Source: CAD feature listing. Evaluate the final solid. Frame: model axes, mm. A direction names the side the tool comes from. Give positions to 0.01 mm unless a question says otherwise; leave off trailing zeros. Order: outer loops, then holes, each group sorted by start corner. A loop starts at its lowest first (then second) coordinate and runs counter-clockwise, first axis right, second up.
from build123d import *

# Parameters (mm, degrees)
EXTRUDE_1_DEPTH        = 180
HOLE_WIZARD_M6_1_D     = 5
HOLE_WIZARD_M6_1_DEPTH = 28
HOLE_WIZARD_M6_1_TIP   = 1.502151548


with BuildPart() as part:
    # 草图1 → 凸台-拉伸1 (new body)
    with BuildSketch(Plane.XY):
        Polygon((12.5, 0), (0, 0), (-3.5, 3.5), (-3.5, 6.2), (2.25, 6.2), (2.25, 9.5), (10.25, 9.5), (10.25, 6.2), (16, 6.2), (16, 3.5), align=None)
    extrude(amount=EXTRUDE_1_DEPTH)

    # M6 螺纹孔1
    with Locations(Plane(origin=(6.25, 9.5, 158), x_dir=(0, 0, 1), z_dir=(0, 1, 0))):
        with Locations((0, 0), (-49, 0), (-136, 0), (-87, 0)):
            Hole(HOLE_WIZARD_M6_1_D / 2, depth=HOLE_WIZARD_M6_1_DEPTH)
            with Locations((0, 0, -(HOLE_WIZARD_M6_1_DEPTH + HOLE_WIZARD_M6_1_TIP / 2))):  # 118° drill point
                Cone(0, HOLE_WIZARD_M6_1_D / 2, HOLE_WIZARD_M6_1_TIP, mode=Mode.SUBTRACT)


solid = part.part
(1) Section A-A, the plane x = 6.25. Return loops of the section in (y, z).
(2) Section B-B, the plane z = 71. Return loops of the section in (x, y), plus the area to 4 significant figures.
(3) Access query for faces 1 (the flat face through (6, 9.5, 89)), 2 (the flat face through (-1, 6.2, 89)), 3 (the flat face through (10.25, 8, 89)). Directions: +Z, -Z, +X, -X, +Y, -Y. A direction counts if a zero-diameter tool reaches every point of the face in a straight line with its end or side. Return the directions, or none.
(4) Section D-D, the plane z = 154. Return loops of the section in (x, y).
(5) Line query: line 1 along Z through (x, y) = (6, 7.25); line 2 along X through (y, z) = (4.5, 158); line 3 along X through (y, z) = (7.75, 166). Output: solid intervals per line, ascending.
(6) Section C-C, the plane y = 1.5. Return loops of the section in (x, z), plus the area to 3 significant figures.
(7) Draft query along Z for faces 4 (the flat face through (6, 4, 0)), 5 (the flat face through (6, 4, 180)), 6 (the cylindrical face through (7.001, 4.684, 155.615)), 7 (the flat face through (14.3, 1.8, 88.7)). Return one class per face: +Z half, -Z half, draft (parallel to the pull), parting line (faces both ways), or undercut.
(8) Pin query (flat end, axial travel): pin 1 Ø1 at (y, z) = (8, 64.5) entering from -X; pin 2 Ø3 at (y, z) = (8, 114) entering from +X. Return the tip coordinate at first contact, or that it passes through.
Checks:
1. outline: (0, 0) - (9.5, 0) - (9.5, 19.5) - (0, 19.5) - close; (0, 24.5) - (9.5, 24.5) - (9.5, 68.5) - (0, 68.5) - close; (0, 73.5) - (9.5, 73.5) - (9.5, 106.5) - (0, 106.5) - close; (0, 111.5) - (9.5, 111.5) - (9.5, 155.5) - (0, 155.5) - close; (0, 160.5) - (9.5, 160.5) - (9.5, 180) - (0, 180) - close
2. outline: (-3.5, 3.5) - (0, 0) - (3.75, 0) - (3.75, 9.5) - (2.25, 9.5) - (2.25, 6.2) - (-3.5, 6.2) - close; (8.75, 0) - (12.5, 0) - (16, 3.5) - (16, 6.2) - (10.25, 6.2) - (10.25, 9.5) - (8.75, 9.5) - close
2. area: 87.55 mm2
3. face 1: +Z, -Z, +X, -X, +Y
3. face 2: +Z, -Z, -X, +Y
3. face 3: +Z, -Z, +X, +Y
4. outline: (-3.5, 3.5) - (0, 0) - (12.5, 0) - (16, 3.5) - (16, 6.2) - (10.25, 6.2) - (10.25, 9.5) - (2.25, 9.5) - (2.25, 6.2) - (-3.5, 6.2) - close
5. line 1: z = 0 to 19.51, 24.49 to 68.51, 73.49 to 106.51, 111.49 to 155.51, 160.49 to 180
5. line 2: x = -3.5 to 3.75, 8.75 to 16
5. line 3: x = 2.25 to 10.25
6. outline: (-1.5, 0) - (14, 0) - (14, 180) - (-1.5, 180) - close; hole circle Ø5 at (6.25, 22); hole circle Ø5 at (6.25, 71); hole circle Ø5 at (6.25, 109); hole circle Ø5 at (6.25, 158)
6. area: 2,710 mm2
7. face 4: -Z half
7. face 5: +Z half
7. face 6: undercut
7. face 7: draft
8. pin 1: stops at x = 2.25
8. pin 2: stops at x = 10.25
